Could you check a few things on this model? Use its own coordinates, in mm. Face numbers are marked on the shaded views. A direction names the side the tool comes from. Coordinates: 2 decimals unless noted, no trailing zeros. Write each loop counter-clockwise with the first axis right and the second up, starting at its lowest first coordinate (ties: lowest second). Pieces come first, ordered by that corner, then holes.
```python
from build123d import *

# Parameters (mm, degrees)
BASE_FLANGE1_DEPTH           = 171.45
SKETCH4_R                    = 4.7625
CUT_EXTRUDE1_DEPTH           = 1.5875
EDGE_FLANGE2_STRIP_W         = 7.8232
EDGE_FLANGE2_STRIP_H         = 1.5875
EDGE_FLANGE2_STRIP_CUT_DEPTH = 164.0078
EDGE_FLANGE2_DEPTH           = 164.0078
EDGE_FLANGE3_STRIP_W         = 7.8232
EDGE_FLANGE3_STRIP_H         = 1.5875
EDGE_FLANGE3_STRIP_CUT_DEPTH = 164.0078
EDGE_FLANGE3_DEPTH           = 164.0078
SKETCH14_R                   = 3.175
CUT_EXTRUDE2_DEPTH           = 1.5875
SKETCH17_R                   = 3.175
CUT_EXTRUDE5_DEPTH           = 1.5875


# Sheet-metal steps are written as plain solids
with BuildPart() as part:
    # Sketch1 → Base-Flange1 (new body)
    with BuildSketch(Plane.XY):
        with BuildLine():
            Line((0, -55.88), (0, -0.7366))
            ThreePointArc((0, -0.7366), (0.215745145, -0.215745145), (0.7366, 0))
            Line((0.7366, 0), (164.7444, 0))
            ThreePointArc((164.7444, 0), (165.265254855, -0.215745145), (165.481, -0.7366))
            Line((165.481, -0.7366), (165.481, -55.88))
            Line((165.481, -55.88), (167.0685, -55.88))
            Line((167.0685, -55.88), (167.0685, -0.7366))
            ThreePointArc((167.0685, -0.7366), (166.38778687, 0.90678687), (164.7444, 1.5875))
            Line((164.7444, 1.5875), (0.7366, 1.5875))
            ThreePointArc((0.7366, 1.5875), (-0.90678687, 0.90678687), (-1.5875, -0.7366))
            Line((-1.5875, -0.7366), (-1.5875, -55.88))
            Line((-1.5875, -55.88), (0, -55.88))
        make_face()
    extrude(amount=BASE_FLANGE1_DEPTH)

    # Sketch4 → Cut-Extrude1 (cut)
    with BuildSketch(Plane(origin=(0, 1.5875, 0), x_dir=(1, 0, 0), z_dir=(0, 1, 0))):
        with Locations(Location((101.981, -97.79, 0), (0, 0, 270))):
            Circle(SKETCH4_R)
    extrude(amount=-CUT_EXTRUDE1_DEPTH, mode=Mode.SUBTRACT)

    # Edge-Flange2 strip (across the edge) → Edge-Flange2 strip cut (cut)
    with BuildSketch(Plane(origin=(164.7444, 0, 171.45), x_dir=(0, 0, -1), z_dir=(-1, 0, 0))):
        with Locations((-3.175, -0.79375)):
            Rectangle(EDGE_FLANGE2_STRIP_W, EDGE_FLANGE2_STRIP_H)
    extrude(amount=EDGE_FLANGE2_STRIP_CUT_DEPTH, mode=Mode.SUBTRACT)

    # Edge-Flange2 section (across the edge) → Edge-Flange2 (add)
    with BuildSketch(Plane(origin=(164.7444, 0, 171.45), x_dir=(0, 0, -1), z_dir=(-1, 0, 0))):
        with BuildLine():
            Line((-1.5875, 0.7366), (-1.5875, 55.88))
            Line((-1.5875, 55.88), (0, 55.88))
            Line((0, 55.88), (0, 0.7366))
            ThreePointArc((0, 0.7366), (0.215745145, 0.215745145), (0.7366, 0))
            Line((0.7366, 0), (0.7366, -1.5875))
            ThreePointArc((0.7366, -1.5875), (-0.90678687, -0.90678687), (-1.5875, 0.7366))
        make_face()
    extrude(amount=EDGE_FLANGE2_DEPTH)

    # Edge-Flange3 strip (across the edge) → Edge-Flange3 strip cut (cut)
    with BuildSketch(Plane(origin=(0.7366, 0, 0), x_dir=(0, 0, 1), z_dir=(1, 0, 0))):
        with Locations((-3.175, -0.79375)):
            Rectangle(EDGE_FLANGE3_STRIP_W, EDGE_FLANGE3_STRIP_H)
    extrude(amount=EDGE_FLANGE3_STRIP_CUT_DEPTH, mode=Mode.SUBTRACT)

    # Edge-Flange3 section (across the edge) → Edge-Flange3 (add)
    with BuildSketch(Plane(origin=(0.7366, 0, 0), x_dir=(0, 0, 1), z_dir=(1, 0, 0))):
        with BuildLine():
            Line((-1.5875, 0.7366), (-1.5875, 55.88))
            Line((-1.5875, 55.88), (0, 55.88))
            Line((0, 55.88), (0, 0.7366))
            ThreePointArc((0, 0.7366), (0.215745145, 0.215745145), (0.7366, 0))
            Line((0.7366, 0), (0.7366, -1.5875))
            ThreePointArc((0.7366, -1.5875), (-0.90678687, -0.90678687), (-1.5875, 0.7366))
        make_face()
    extrude(amount=EDGE_FLANGE3_DEPTH)

    # Sketch14 → Cut-Extrude2 (cut)
    with BuildSketch(Plane(origin=(0, 1.5875, 0), x_dir=(1, 0, 0), z_dir=(0, 1, 0))):
        with Locations(Location((155.956, -158.75, 0), (0, 0, 270))):
            Circle(SKETCH14_R)
        with Locations(Location((9.525, -158.75, 0), (0, 0, 270))):
            Circle(SKETCH14_R)
    extrude(amount=-CUT_EXTRUDE2_DEPTH, mode=Mode.SUBTRACT)

    # Sketch17 → Cut-Extrude5 (cut)
    with BuildSketch(Plane.XY.offset(173.0375)):
        with Locations((86.106, -19.7866)):
            Circle(SKETCH17_R)
    extrude(amount=-CUT_EXTRUDE5_DEPTH, mode=Mode.SUBTRACT)


solid = part.part
```
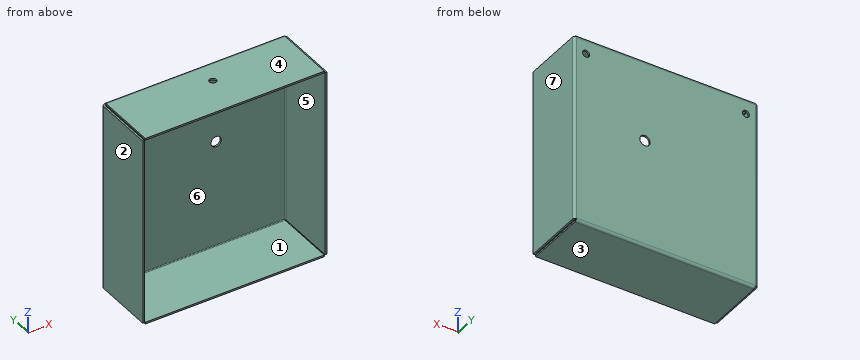
1. On a 3-axis mill with a long thin cutter (end or side, diameter ignored), from which of +Z, -Z, +X, -X, +Y, -Y can I reach the whole of each face in a straight line? I mean the marked faces 5, 6 and 7. Say none if no direction works.
Verdict:
face 5: +Z, -Z, -Y
face 6: -Y
face 7: +Z, -Z, +X, +Y, -Y
2. I want a section at B-B on z = 97.79. Please give me the cut outline in (x, y), plus the area to 3 significant figures.
Verdict:
outline: (-1.59, -55.88) - (0, -55.88) - (0, -0.74) arc R0.74 cw to (0.74, 0) - (97.22, 0) - (97.22, 1.59) - (0.74, 1.59) arc R2.32 ccw to (-1.59, -0.74) - close; (106.74, 0) - (164.74, 0) arc R0.74 cw to (165.48, -0.74) - (165.48, -55.88) - (167.07, -55.88) - (167.07, -0.74) arc R2.32 ccw to (164.74, 1.59) - (106.74, 1.59) - close
area: 428 mm2
3. I want a section at A-A on y = -35. Please give me the cut outline in (x, z).
Verdict:
outline: (-1.59, 0) - (0, 0) - (0, 171.45) - (-1.59, 171.45) - close; (0.74, -1.59) - (164.74, -1.59) - (164.74, 0) - (0.74, 0) - close; (0.74, 171.45) - (164.74, 171.45) - (164.74, 173.04) - (0.74, 173.04) - close; (165.48, 0) - (167.07, 0) - (167.07, 171.45) - (165.48, 171.45) - close
4. For pin 1 (2 mm diameter, centred on x = 41, z = 51, fed in from -Y); pin 2 (4 mm diameter, centred on x = 155.956, z = 158.75, fed in from +Y), each with a flat end and sliding along its axis, tell me the tip position at first contact or that it passes through.
Verdict:
pin 1: stops at y = 0
pin 2: passes through
5. Please list where these lines run through material, in increasing order: line 1 along Z through (x, y) = (144.5, -2); line 2 along X through (y, z) = (-9, 7); line 3 along Y through (x, z) = (56, 46).
Verdict:
line 1: z = -1.59 to 0, 171.45 to 173.04
line 2: x = -1.59 to 0, 165.48 to 167.07
line 3: y = 0 to 1.59
6. If we mould it in two halves opening along Z, with no side actions, what happens to the marked faces 1, 2, 3 and 4? For each: pulls with the +Z half, pulls with the -Z half, needs draft (parallel to the pull), parting line crosses it, or undercut.
Verdict:
face 1: undercut
face 2: needs draft
face 3: pulls with the -Z half
face 4: pulls with the +Z half
7. I want a section at C-C on z = 158.75. Please give me the cut outline in (x, y), plus the area to 3 significant figures.
Verdict:
outline: (-1.59, -55.88) - (0, -55.88) - (0, -0.74) arc R0.74 cw to (0.74, 0) - (6.35, 0) - (6.35, 1.59) - (0.74, 1.59) arc R2.32 ccw to (-1.59, -0.74) - close; (12.7, 0) - (152.78, 0) - (152.78, 1.59) - (12.7, 1.59) - close; (159.13, 0) - (164.74, 0) arc R0.74 cw to (165.48, -0.74) - (165.48, -55.88) - (167.07, -55.88) - (167.07, -0.74) arc R2.32 ccw to (164.74, 1.59) - (159.13, 1.59) - close
area: 423 mm2
8. I want a section at D-D on x = 110.5. Please give me the cut outline in (y, z), plus the area to 3 significant figures.
Verdict:
outline: (-55.88, -1.59) - (-0.74, -1.59) arc R2.32 ccw to (1.59, 0.74) - (1.59, 170.71) arc R2.32 ccw to (-0.74, 173.04) - (-55.88, 173.04) - (-55.88, 171.45) - (-0.74, 171.45) arc R0.74 cw to (0, 170.71) - (0, 0.74) arc R0.74 cw to (-0.74, 0) - (-55.88, 0) - close
area: 453 mm2
